Design review of the part built by this model. Coordinates are the model's own, in mm. Face numbers are marked on the shaded views. Give positions to 0.01 mm unless a question says otherwise; leave off trailing zeros. Order: outer loops, then holes, each group sorted by start corner. A loop starts at its lowest first (then second) coordinate and runs counter-clockwise, first axis right, second up. Notation, with made-up numbers: (11.25, 46.25) -> (32.25, 46.25) arc R14 cw to (32.25, 72.25) -> close; hole circle Ø2 at (14, -39.75). An arc over 180 degrees is marked (long way). One line per item, written item: value. Start each with the question number.
1) The part is to be moulded in two halves that separate along Z. For the marked faces 1, 2 and 3, say which applies: released by +Z, released by -Z, zero draft, split by the parting line, or undercut.
2) Consider section B-B (z = 0). State the section outline as (x, y) points.
3) Wall thickness on line 1 along X through (y, z) = (2.4, -2); line 2 along X through (y, z) = (3.5, -1.5); line 3 along Z through (x, y) = (-2.25, 1.25): over which ranges is each line inside the solid? List them lowest first. Write a range as from..to.
4) For pin 1 (4 mm diameter, centred on x = -2, z = -4.5, fed in from -Y); pin 2 (1.5 mm diameter, centred on y = 0.5, z = -1, fed in from -X); pin 3 (2 mm diameter, centred on x = -3.5, y = 1, fed in from +Z), all flat-tipped, find the tip position at first contact; note any pin that passes through.
5) Consider section C-C (y = 1.7). State the section outline as (x, z) points, plus the area to 3 significant figures.
6) Consider section A-A (x = 0). State the section outline as (y, z) points, plus the area to 3 significant figures.
7) Consider section D-D (y = 0.55). State the section outline as (x, z) points, plus the area to 3 significant figures.
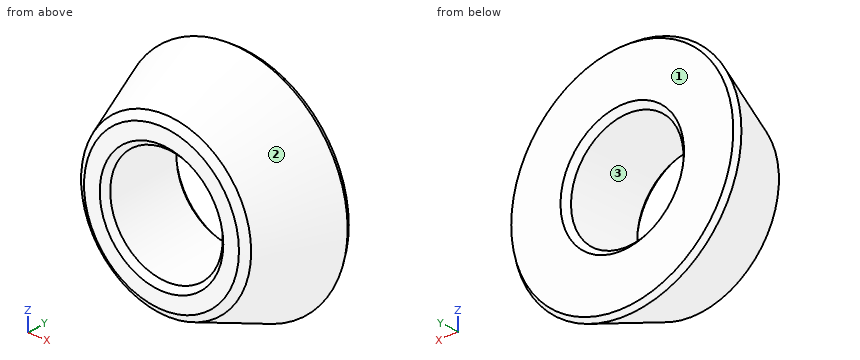
from build123d import *

# Parameters (mm, degrees)
CHAMFER3_SIZE = 0.3


with BuildPart() as part:
    # Sketch3 → Revolve1 (revolve)
    with BuildSketch(Plane.XY):
        Polygon((3.05, 4.6), (3.05, 0), (4.5, 0), (6.31983867, 4.6), align=None)
    revolve(axis=Axis((0, 4.6, 0), (0, -1, 0)))

    # Chamfer3
    chamfer3_edges = [part.edges().sort_by_distance(p)[0] for p in [
        (-6.31983867, 4.6, 0),
        (-4.5, 0, 0),
        (-3.05, 0, 0),
        (-3.05, 4.6, 0),
    ]]
    chamfer(chamfer3_edges, length=CHAMFER3_SIZE)


solid = part.part
Checked values:
1. face 1: zero draft
1. face 2: split by the parting line
1. face 3: undercut
2. outline: (-6.21, 4.32) -> (-4.61, 0.28) -> (-4.2, 0) -> (-3.35, 0) -> (-3.05, 0.3) -> (-3.05, 4.3) -> (-3.35, 4.6) -> (-6.02, 4.6) -> close; (3.05, 0.3) -> (3.35, 0) -> (4.2, 0) -> (4.61, 0.28) -> (6.21, 4.32) -> (6.02, 4.6) -> (3.35, 4.6) -> (3.05, 4.3) -> close
3. line 1: x = -5.07..-2.3, 2.3..5.07
3. line 2: x = -5.69..-2.66, 2.66..5.69
3. line 3: z = -4.46..-2.06, 2.06..4.46
4. pin 1: stops at y = 0
4. pin 2: stops at x = -4.92
4. pin 3: stops at z = 4.37
5. outline: circle Ø10.35 at (0, 0); hole circle Ø6.1 at (0, 0)
5. area: 54.8 mm^2
6. outline: (0, -4.2) -> (0.28, -4.61) -> (4.32, -6.21) -> (4.6, -6.02) -> (4.6, -3.35) -> (4.3, -3.05) -> (0.3, -3.05) -> (0, -3.35) -> close; (0, 3.35) -> (0.3, 3.05) -> (4.3, 3.05) -> (4.6, 3.35) -> (4.6, 6.02) -> (4.32, 6.21) -> (0.28, 4.61) -> (0, 4.2) -> close
6. area: 21.4 mm^2
7. outline: circle Ø9.44 at (0, 0); hole circle Ø6.1 at (0, 0)
7. area: 40.7 mm^2
